```python
from build123d import *

# Parameters (mm, degrees)
SKETCH1_R           = 50
BOSS_EXTRUDE1_DEPTH = 10
BOSS_EXTRUDE2_DEPTH = 180
SKETCH3_R           = 50
BOSS_EXTRUDE3_DEPTH = 10


with BuildPart() as part:
    # Sketch1 → Boss-Extrude1 (new body)
    with BuildSketch(Plane(origin=(0, 0, 0), x_dir=(0, 1, 0), z_dir=(0, 0, 1))):
        with Locations(Location((0, 0, 0), (0, 0, 270))):
            Circle(SKETCH1_R)
    extrude(amount=BOSS_EXTRUDE1_DEPTH)

    # Sketch2 → Boss-Extrude2 (add)
    with BuildSketch(Plane.XY.offset(10)):
        with BuildLine():
            Line((0, 50), (0, 45))
            ThreePointArc((0, 45), (-45, 0), (0, -45))
            Line((0, -45), (0, -50))
            ThreePointArc((0, -50), (-50, 0), (0, 50))
        make_face()
    extrude(amount=BOSS_EXTRUDE2_DEPTH)

    # Sketch3 → Boss-Extrude3 (add)
    with BuildSketch(Plane.XY.offset(190)):
        Circle(SKETCH3_R)
    extrude(amount=BOSS_EXTRUDE3_DEPTH)


solid = part.part
```
Part model, mm, in its own coordinate system. A direction names the side the tool comes from. Round coordinates to 2 decimals unless told otherwise and drop trailing zeros. Loops run counter-clockwise (first coordinate to the right, second up) from the corner with the lowest first, then second, coordinate; pieces in that order, holes last. Notation, with made-up numbers: (40, 84) -> (83, 84) arc R26 ccw to (83, 99) -> close; hole circle Ø8 at (-21, -17). An arc over 180 degrees is marked (long way). Use one line per item in the form item = value. Start each with the question number.
Item 1: Tool access for faces 3 (the flat face through (0, 48, 99)), 4 (the cylindrical face through (-44.99, 0.99, 98.74)), 5 (the flat face through (-1, 1, 0)): list every direction of +Z, -Z, +X, -X, +Y, -Y with a clear straight run to the whole face (end or side of a thin tool).
Item 2: Drill centre lines: line 1 along Z through (x, y) = (-32, 15); line 2 along Y through (x, z) = (-32.5, 182.5); line 3 along Y through (x, z) = (-25.5, 147). Where is each one in solid material? Low to high.
Item 3: Band-saw the part on A-A (y = 0). List the corners of the cut face in (x, z), plus the area to 3 significant figures.
Item 4: Band-saw the part on C-C (z = 117). List the corners of the cut face in (x, y), plus the area to 3 significant figures.
Item 5: Drop flat-ended pins along their axis: pin 1 Ø8 at (x, z) = (-34, 70.5) entering from -Y; pin 2 Ø4 at (x, z) = (-38.5, 39) entering from -Y; pin 3 Ø8 at (y, z) = (-20, 33.5) entering from -X. Give the stop position or say it passes through.
Item 6: Two-plate mould, pull along Y, no slides. Class faces 1 (the flat face through (2, 1, 190)), 2 (the flat face through (0, -47, 99)): released by +Y, released by -Y, zero draft, split by the parting line, or undercut.
Item 7: Band-saw the part on B-B (x = 19). List the corners of the cut face in (y, z), plus the area to 3 significant figures.
Item 8: Band-saw the part on D-D (x = -13). List the corners of the cut face in (y, z).
Data:
q1.face_3 = +X, +Y, -Y
q1.face_4 = +X
q1.face_5 = -Z, +X, -X, +Y, -Y
q2.line_1 = 0 to 10, 190 to 200
q2.line_2 = -38 to -31.12, 31.12 to 38
q2.line_3 = -43.01 to -37.08, 37.08 to 43.01
q3.outline = (-50, 0) -> (50, 0) -> (50, 10) -> (-45, 10) -> (-45, 190) -> (50, 190) -> (50, 200) -> (-50, 200) -> close
q3.area = 2,900 mm^2
q4.outline = (0, -50) -> (0, -45) arc R45 cw to (0, 45) -> (0, 50) arc R50 ccw to start
q4.area = 746 mm^2
q5.pin_1 = -40
q5.pin_2 = -34.17
q5.pin_3 = -47.37
q6.face_1 = undercut
q6.face_2 = zero draft
q7.outline = (-46.25, 0) -> (46.25, 0) -> (46.25, 10) -> (-46.25, 10) -> close; (-46.25, 190) -> (46.25, 190) -> (46.25, 200) -> (-46.25, 200) -> close
q7.area = 1,850 mm^2
q8.outline = (-48.28, 0) -> (48.28, 0) -> (48.28, 200) -> (-48.28, 200) -> close; hole (-43.08, 10) -> (43.08, 10) -> (43.08, 190) -> (-43.08, 190) -> close
